```python
from build123d import *

# Parameters (mm, degrees)
BOSS_EXTRUDE1_DEPTH = 16
SKETCH2_R           = 1.625
CUT_EXTRUDE1_DEPTH  = 21.322401433
CHAMFER1_SIZE       = 1.7
FILLET1_SIZE        = 4
FILLET1_SIZE_2      = 6


with BuildPart() as part:
    # Sketch1 → Boss-Extrude1 (new body)
    with BuildSketch(Plane.XY):
        Polygon((-4, -8), (-4, 8), (0, 8), (0, 3), (6, 3), (6, -3), (0, -3), (0, -8), align=None)
    extrude(amount=BOSS_EXTRUDE1_DEPTH)

    # Sketch2 → Cut-Extrude1 (cut, through all)
    with BuildSketch(Plane.XZ.offset(3)):
        with Locations(Location((3.25, 12, 0), (0, 0, 270))):
            Circle(SKETCH2_R)
        with Locations(Location((3.25, 4, 0), (0, 0, 270))):
            Circle(SKETCH2_R)
    extrude(amount=-CUT_EXTRUDE1_DEPTH, mode=Mode.SUBTRACT)

    # Chamfer1
    chamfer1_edges = [part.edges().sort_by_distance(p)[0] for p in [
        (6, 0, 0),
    ]]
    chamfer(chamfer1_edges, length=CHAMFER1_SIZE)

    # Fillet1
    # an asymmetric fillet: 6, 4 mm, written as the material it takes off along each edge
    with BuildSketch(Plane(origin=(6, 18, 16), x_dir=(0, 0, -1), z_dir=(0, -1, 0))) as fillet1_piece_1:
        with BuildLine():
            Bezier((FILLET1_SIZE, 0), (0, 0), (0, -FILLET1_SIZE_2), weights=[1, 0.707106781, 1])
            Line((0, -FILLET1_SIZE_2), (0, 0))
            Line((0, 0), (FILLET1_SIZE, 0))
        make_face()
    extrude(amount=36, mode=Mode.SUBTRACT)


solid = part.part
```
Check sheet for the modelled part. Datum: model origin and axes. Units: mm. A direction names the side the tool comes from. Coordinates: 2 decimals unless noted, no trailing zeros. Order: outer loops, then holes, each group sorted by start corner. A loop starts at its lowest first (then second) coordinate and runs counter-clockwise, first axis right, second up. Notation, with made-up numbers: M 60.25,72 L 66.25,72 A33 ccw 66.25,102 Z; hole C 6,-9.75 d2. An arc over 180 degrees is marked long. Write each question's results on one line, items separated by ' | '. Start each with the question number.
1. Mould release check, pull along X, two halves, no side actions. Record for faces 4 (the face through (0, 6, 8)), 5 (the face through (3.321, -0.042, 13.623)), 6 (the face through (3, -3, 8)): +X half, -X half, draft (parallel to the pull), parting line (faces both ways), or undercut.
2. Cross-section at B-B on z = 1. Record the cut outline in (x, y).
3. Cross-section at C-C on y = 2.25. State how many separate pieces and enclosed holes the cut face has, and give its area (3 significant figures).
4. Cross-section at A-A on z = 4. Record the cut outline in (x, y) (3 decimals), and give its area (3 significant figures).
5. Material ranges on probe 1 along X at (y, z) = (-1.2, 4) (3 decimals); probe 2 along Y at (x, z) = (3.5, 10); probe 3 along Z at (x, y) = (4, 2), recorded low to high.
6. Go/stop test with flat-tipped pins: P1, Ø5, axis at x = 3.25, z = 4, coming from the +Y side; P2, Ø1.8, axis at x = 2, z = 10, coming from the -Y side; P3, Ø1.5, axis at y = -5, z = 4, coming from the +X side. Record where each tip stops, or that it passes through.
7. Access from +Z, -Z, +X, -X, +Y, -Y to the whole of each face (thin tool, end or side, straight path). Record for faces 1 (the face through (0, -5, 8)), 2 (the face through (3, 3, 8)), 3 (the face through (3.321, -0.042, 5.623)).
Checks:
1) face 4: +X half | face 5: undercut | face 6: draft
2) outline: M -4,-8 L 0,-8 L 0,-3 L 5.3,-3 L 5.3,3 L 0,3 L 0,8 L -4,8 Z
3) separate pieces: 1 | enclosed holes: 2 | area: 137 mm²
4) outline: M -4,-8 L 0,-8 L 0,-3 L 1.625,-3 L 1.625,3 L 0,3 L 0,8 L -4,8 Z; M 4.875,-3 L 6,-3 L 6,3 L 4.875,3 Z | area: 80.5 mm²
5) probe 1: x = -4 to 1.625, 4.875 to 6 | probe 2: y = -3 to 3 | probe 3: z = 0 to 2.56, 5.44 to 10.56, 13.44 to 14.98
6) P1: stops at y = 3 | P2: stops at y = -3 | P3: stops at x = 0
7) face 1: +Z, -Z, +X, -Y | face 2: +Z, -Z, +X, +Y | face 3: +Y, -Y
